Work out the finished part from the listing and answer in its coordinate system (mm). A direction names the side the tool comes from. Give positions to 0.01 mm unless a question says otherwise; leave off trailing zeros. Loops run counter-clockwise (first coordinate to the right, second up) from the corner with the lowest first, then second, coordinate; pieces in that order, holes last. Notation, with made-up numbers: (-30, -1.5) - (11, -1.5) arc R23 cw to (11, 28.5) - close; hole circle Ø5 at (78.5, 78.5). An arc over 180 degrees is marked (long way). Use CSV: the item, a comma, the result in double quotes.
from build123d import *

# Parameters (mm, degrees)
SKETCH1_R           = 22.482
SKETCH1_R_2         = 19.45
SKETCH1_R_3         = 5
SKETCH1_R_4         = 2.8
BOSS_EXTRUDE1_DEPTH = 19.05
SKETCH1_5_R         = 2
BOSS_EXTRUDE3_DEPTH = 6.35
CHAMFER1_SIZE       = 4.7625
SHELL1_START        = -959.849406281
SHELL1_OUTLINE_R    = 20.481999936
SHELL1_DEPTH        = 13.459072749
SHELL1_2_DEPTH      = 4.349999936


with BuildPart() as part:
    # Sketch1 → Boss-Extrude1 (new body)
    # profile 1 of 6: a face of its own
    with BuildSketch(Plane.XY.offset(-959.849406281)):
        with Locations(Location((-167.581326331, 1325.789589838, 0), (0, 0, 180))):
            Circle(SKETCH1_R)
        with Locations((-167.581326331, 1325.789589838)):
            Circle(SKETCH1_R_2, mode=Mode.SUBTRACT)
    # profile 2 of 6: a face of its own
    with BuildSketch(Plane.XY.offset(-959.849406281)):
        with Locations((-167.581326331, 1325.789589838)):
            Circle(SKETCH1_R_2)
        with Locations((-158.719406684, 1324.967166478)):
            Circle(SKETCH1_R_3, mode=Mode.SUBTRACT)
        with Locations((-176.443245977, 1326.612013197)):
            Circle(SKETCH1_R_3, mode=Mode.SUBTRACT)
        with Locations((-168.704072827, 1313.691575939)):
            Circle(SKETCH1_R_4, mode=Mode.SUBTRACT)
        Polygon((-169.416951474, 1318.076211503), (-167.966159705, 1333.709036048), (-165.745701187, 1333.502968172), (-167.196492956, 1317.870143628), align=None, mode=Mode.SUBTRACT)
    # profile 3 of 6: a face of its own
    with BuildSketch(Plane.XY.offset(-959.849406281)):
        with Locations((-168.704072827, 1313.691575939)):
            Circle(SKETCH1_R_4)
    # profile 4 of 6: a face of its own
    with BuildSketch(Plane.XY.offset(-959.849406281)):
        with Locations((-158.719406684, 1324.967166478)):
            Circle(SKETCH1_R_3)
    # profile 5 of 6: a face of its own
    with BuildSketch(Plane.XY.offset(-959.849406281)):
        Polygon((-167.966159705, 1333.709036048), (-165.745701187, 1333.502968172), (-167.196492956, 1317.870143628), (-169.416951474, 1318.076211503), align=None)
    # profile 6 of 6: a face of its own
    with BuildSketch(Plane.XY.offset(-959.849406281)):
        with Locations((-176.443245977, 1326.612013197)):
            Circle(SKETCH1_R_3)
    extrude(amount=BOSS_EXTRUDE1_DEPTH)

    # Sketch1<5> → Boss-Extrude3 (add)
    # profile 1 of 2: a face of its own
    with BuildSketch(Plane.XY.offset(-959.849406281)):
        with BuildLine():
            ThreePointArc((-187.111667422, 1336.925392497), (-181.91942666, 1343.106032976), (-174.878765823, 1347.054295358))
            ThreePointArc((-174.878765823, 1347.054295358), (-176.443944893, 1347.205674138), (-177.935770468, 1347.702823524))
            ThreePointArc((-177.935770468, 1347.702823524), (-186.383740435, 1348.497684162), (-187.178601073, 1340.049714195))
            ThreePointArc((-187.178601073, 1340.049714195), (-186.968441908, 1338.4913387), (-187.111667422, 1336.925392497))
        make_face()
        with Locations((-184.151583548, 1345.801858569)):
            Circle(SKETCH1_5_R, mode=Mode.SUBTRACT)
    # profile 2 of 2: a face of its own
    with BuildSketch(Plane.XY.offset(-959.849406281)):
        with BuildLine():
            ThreePointArc((-147.984051588, 1311.529465481), (-148.194210754, 1313.087840976), (-148.050985239, 1314.653787179))
            ThreePointArc((-148.050985239, 1314.653787179), (-153.243226001, 1308.4731467), (-160.283886838, 1304.524884318))
            ThreePointArc((-160.283886838, 1304.524884318), (-158.718707768, 1304.373505537), (-157.226882193, 1303.876356151))
            ThreePointArc((-157.226882193, 1303.876356151), (-148.778912226, 1303.081495514), (-147.984051588, 1311.529465481))
        make_face()
        with Locations((-151.011069114, 1305.777321107)):
            Circle(SKETCH1_5_R, mode=Mode.SUBTRACT)
    extrude(amount=BOSS_EXTRUDE3_DEPTH)

    # Chamfer1
    chamfer1_edges = [part.edges().sort_by_distance(p)[0] for p in [
        (-145.099326331, 1325.789589838, -940.799406281),
    ]]
    chamfer(chamfer1_edges, length=CHAMFER1_SIZE)

    # Shell1: read off the stored shape, not the designer's step
    # Shell1 outline → Shell1 (cut)
    with BuildSketch(Plane.XY.offset(SHELL1_START)):
        with Locations((-167.581326331, 1325.789589838)):
            Circle(SHELL1_OUTLINE_R)
    extrude(amount=SHELL1_DEPTH, mode=Mode.SUBTRACT)

    # Shell1 2 outline → Shell1 2 (cut)
    with BuildSketch(Plane.XY.offset(SHELL1_START)):
        with BuildLine():
            ThreePointArc((-179.248478566, 1346.124035779), (-179.779181822, 1346.754235772), (-180.427741548, 1347.262338379))
            ThreePointArc((-180.427741548, 1347.262338379), (-181.600547064, 1342.720914984), (-186.281027509, 1342.415788733))
            ThreePointArc((-186.281027509, 1342.415788733), (-185.902815813, 1341.683836624), (-185.382666181, 1341.044898178))
            ThreePointArc((-185.382666181, 1341.044898178), (-184.97132452, 1338.625607411), (-185.229107011, 1336.185173441))
            ThreePointArc((-185.229107011, 1336.185173441), (-180.643908398, 1341.565561159), (-174.502685337, 1345.066703493))
            ThreePointArc((-174.502685337, 1345.066703493), (-176.948372758, 1345.268651042), (-179.248478566, 1346.124035779))
        make_face()
        with BuildLine():
            ThreePointArc((-149.77998648, 1310.534281498), (-150.191328141, 1312.953572265), (-149.93354565, 1315.394006235))
            ThreePointArc((-149.93354565, 1315.394006235), (-154.518744264, 1310.013618517), (-160.659967324, 1306.512476183))
            ThreePointArc((-160.659967324, 1306.512476183), (-158.214279903, 1306.310528634), (-155.914174095, 1305.455143896))
            ThreePointArc((-155.914174095, 1305.455143896), (-155.383470839, 1304.824943903), (-154.734911113, 1304.316841296))
            ThreePointArc((-154.734911113, 1304.316841296), (-153.562105598, 1308.858264691), (-148.881625153, 1309.163390942))
            ThreePointArc((-148.881625153, 1309.163390942), (-149.259836848, 1309.895343052), (-149.77998648, 1310.534281498))
        make_face()
    extrude(amount=SHELL1_2_DEPTH, mode=Mode.SUBTRACT)

    # Shell1 3 outline → Shell1 3 (revolve, cut)
    with BuildSketch(Plane(origin=(-167.581326331, 1325.789589838, 0), x_dir=(1, 0, 0), z_dir=(0, -1, 0))):
        Polygon((16.891072849, -942.799406345), (0, -942.799406345), (0, -946.390333532), (20.481999936, -946.390333532), align=None)
    revolve(axis=Axis((-167.581326331, 1325.789589838, 0), (0, 0, 1)), mode=Mode.SUBTRACT)


solid = part.part
Item 1: For faces 5 (the flat face through (-151, 1308, -953.499)), 6 (the cylindrical face through (-189.025, 1319.037, -952.806)), 7 (the cylindrical face through (-176.42, 1347.2, -956.72)), 8 (the cylindrical face through (-156.57, 1343.06, -953.21)), 9 (the cylindrical face through (-158.74, 1304.38, -956.72)), determine the directions among +Z, -Z, +X, -X, +Y, -Y from which every point of the face is accessible in a straight line to the end or side of a thin tool.
Determined:
face 5,"+Z, +X, -Y"
face 6,"+Z"
face 7,"+Z, -Z, +Y"
face 8,"-Z"
face 9,"+Z, -Z, -Y"
Item 2: A cutting plane is placed at B-B on z = -950. Determine the outline of the cut face in (x, y), and give its area (3 significant figures).
Determined:
outline,"circle Ø44.96 at (-167.58, 1325.79); hole circle Ø40.96 at (-167.58, 1325.79)"
area,"270 mm²"
Item 3: Find the intervals of material crossed by line 1 (Y direction, x = -167, z = -950.75); line 2 (Y direction, x = -182.5, z = -956.25); line 3 (X direction, y = 1323.5, z = -951.5), in increasing order.
Determined:
line 1,"y = 1303.32 to 1305.32, 1346.26 to 1348.26"
line 2,"y = 1308.97 to 1311.76, 1342.16 to 1344.67, 1346.93 to 1349.88"
line 3,"x = -189.95 to -187.93, -147.23 to -145.22"
Item 4: Given P1, Ø3, axis at x = -184.15, y = 1345.8, coming from the -Z side; P2, Ø4, axis at x = -166, z = -947.5, coming from the +Y side; P3, Ø5, axis at y = 1310, z = -943, coming from the +X side; P4, Ø1, axis at x = -183.5, z = -946, coming from the +Y side, each flat-ended and moving along its own axis, determine where each tip first touches the part or whether it passes through.
Determined:
P1,"passes through"
P2,"stops at y = 1348.27"
P3,"stops at x = -150.95"
P4,"stops at y = 1342.15"
Item 5: The mould has two halves that part along X. Classify faces 1 (the cylindrical face through (-150.19, 1312.92, -957.7)), 2 (the flat face through (-188, 1331, -959.849)), 3 (the flat face through (-181, 1342, -955.499)), 4 (the conical face through (-165.24, 1307.99, -941.03)): pulls with the +X half, pulls with the -X half, needs draft (parallel to the pull), parting line crosses it, or undercut.
Determined:
face 1,"undercut"
face 2,"needs draft"
face 3,"undercut"
face 4,"parting line crosses it"
Item 6: A cutting plane is placed at A-A on z = -958.25. Determine the outline of the cut face in (x, y), and give its area (3 significant figures).
Determined:
outline,"(-187.18, 1340.05) arc R7 cw to (-187.11, 1336.93) arc R22.48 ccw to (-160.28, 1304.52) arc R7 cw to (-157.23, 1303.88) arc R6 ccw to (-147.98, 1311.53) arc R7 cw to (-148.05, 1314.65) arc R22.48 ccw to (-174.88, 1347.05) arc R7 cw to (-177.94, 1347.7) arc R6 ccw to start; hole (-186.28, 1342.42) arc R4 ccw to (-185.38, 1341.04) arc R9 cw to (-185.23, 1336.19) arc R20.48 ccw to (-160.66, 1306.51) arc R9 cw to (-155.91, 1305.46) arc R4 ccw to (-154.73, 1304.32) arc R4 cw to (-148.88, 1309.16) arc R4 ccw to (-149.78, 1310.53) arc R9 cw to (-149.93, 1315.39) arc R20.48 ccw to (-174.5, 1345.07) arc R9 cw to (-179.25, 1346.12) arc R4 ccw to (-180.43, 1347.26) arc R4 cw to start; hole circle Ø4 at (-184.15, 1345.8); hole circle Ø4 at (-151.01, 1305.78)"
area,"342 mm²"
